Verification items for this drawing (mm, ordinates from the low corner). Coordinates: 2 decimals unless noted, no trailing zeros. Loops run counter-clockwise (first coordinate to the right, second up) from the corner with the lowest first, then second, coordinate; pieces in that order, holes last. Notation, with made-up numbers: M -7.75,24.25 L 23.25,24.25 A30 ccw 23.25,49.25 Z; hole C 37.5,75 d4. An arc over 180 degrees is marked long. Write each question's results on one line, items separated by ' | '. Start each with the question number.
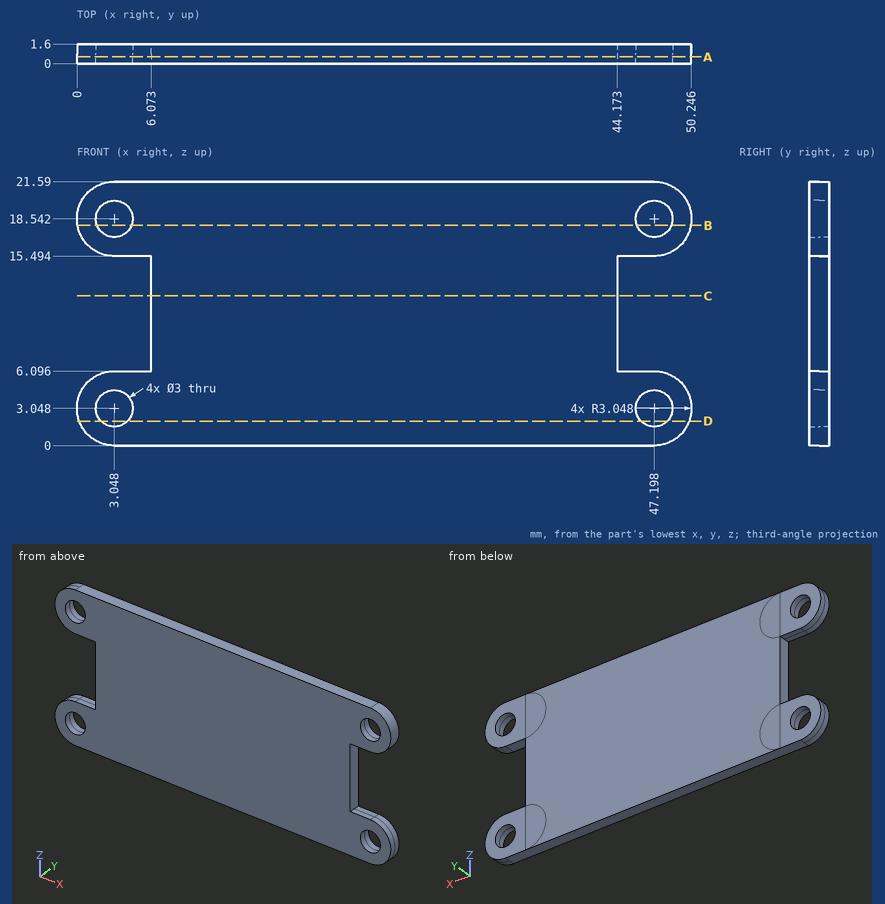
Item 1: Section check D-D (z = 2). Record the cut outline in (x, y), plus the area to 3 significant figures.
Item 2: Section check C-C (z = 12.25). Record the cut outline in (x, y).
Item 3: Section check B-B (z = 18). Record the cut outline in (x, y).
Item 4: Depth check by flat-ended pin: P1, Ø0.8, axis at y = 1, z = 12.5, coming from the -X side. Enter the tip coordinate at first touch or a pass-through.
Item 5: Section check A-A (y = 0.55). Record the cut outline in (x, z), plus the area to 3 significant figures.
Item 6: Thickness scan on line 1 (X direction, y = 0.3, z = 3.75); line 2 (X direction, y = 0.9, z = 19); line 3 (X direction, y = 0.1, z = 12.5). Record the ranges inside material, lowest first.
Computed values:
1) outline: M 0.19,0 L 1.97,0 L 1.97,1.6 L 0.19,1.6 Z; M 4.12,0 L 46.12,0 L 46.12,1.6 L 4.12,1.6 Z; M 48.27,0 L 50.06,0 L 50.06,1.6 L 48.27,1.6 Z | area: 72.9 mm²
2) outline: M 6.07,0 L 44.17,0 L 44.17,1.6 L 6.07,1.6 Z
3) outline: M 0.05,0 L 1.65,0 L 1.65,1.6 L 0.05,1.6 Z; M 4.45,0 L 45.8,0 L 45.8,1.6 L 4.45,1.6 Z; M 48.6,0 L 50.2,0 L 50.2,1.6 L 48.6,1.6 Z
4) P1: stops at x = 6.07
5) outline: M 3.05,0 L 47.2,0 A3.05 ccw 47.2,6.1 L 44.17,6.1 L 44.17,15.49 L 47.2,15.49 A3.05 ccw 47.2,21.59 L 3.05,21.59 A3.05 ccw 3.05,15.49 L 6.07,15.49 L 6.07,6.1 L 3.05,6.1 A3.05 ccw Z; hole C 3.05,3.05 d3; hole C 3.05,18.54 d3; hole C 47.2,3.05 d3; hole C 47.2,18.54 d3 | area: 926 mm²
6) line 1: x = 0.08 to 1.72, 4.37 to 45.87, 48.52 to 50.16 | line 2: x = 0.03 to 1.62, 4.48 to 45.77, 48.63 to 50.21 | line 3: x = 6.07 to 44.17
